Could you check a few things on this model? Use its own coordinates, in mm. Face numbers are marked on the shaded views. A direction names the side the tool comes from. Give positions to 0.01 mm unless a question says otherwise; leave off trailing zeros. Loops run counter-clockwise (first coordinate to the right, second up) from the corner with the lowest first, then second, coordinate; pieces in that order, holes last.
1. For the marked faces 1 and 2, which set-ups out of +Z, -Z, +X, -X, +Y, -Y let a thin tool reach every point of the face, with its end or its side?
2. I need wall thicknesses on line 1 along Z through (x, y) = (2.5, 0.75); line 2 along Y through (x, z) = (-2, 3.25); line 3 along Y through (x, z) = (-3.25, 1.5). Which ranges of each line are inside material? Lowest first, please.
3. For P1, Ø10, axis at y = 5, z = 2.5, coming from the +X side; P2, Ø3, axis at x = 4, y = -2.5, coming from the -Z side; P3, Ø1, axis at y = -6.5, z = 3, coming from the -X side; P4, Ø6, axis at x = 3, y = -2.5, coming from the +Z side, each with a flat end and sliding along its axis, tell me the tip position at first contact or that it passes through.
4. Imagine slicing it at A-A (z = 5.75). List the corners of the cut face in (x, y) for me, plus the area to 3 significant figures.
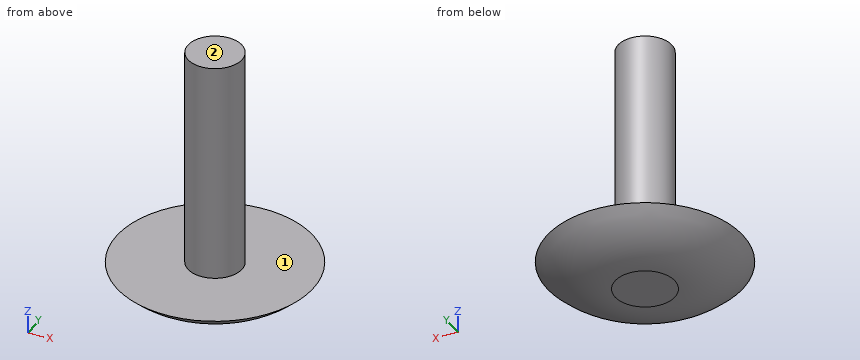
```python
from build123d import *

# Parameters (mm, degrees)
F0_R     = 9.25
F1_DEPTH = 2.7
F2_R     = 2.55
F3_DEPTH = 21


# Not quite as in the source:
# - a fillet or chamfer that OpenCascade refuses, or shapes differently, is made with other operations: its cross-section is extruded or revolved along the edge and cut away or added


with BuildPart() as f1:
    # F0 (on Top) → F1 (new body)
    with BuildSketch(Plane.XY):
        Circle(F0_R)
    extrude(amount=F1_DEPTH)

    # F2 (on face) → F3 (join)
    with BuildSketch(Plane.XY.offset(2.7)):
        Circle(F2_R)
    extrude(amount=F3_DEPTH)

    # F4: fillet of radius 9 on 1 edges, made by hand

    # F4_s1 → F4_t2 (revolve, cut)
    with BuildSketch(Plane.XZ):
        with BuildLine():
            ThreePointArc((9.25, 2.7), (6.3083994259, 0.7024099884), (2.8227144143, 0))
            Line((2.8227144143, 0), (9.25, 0))
            Line((9.25, 0), (9.25, 2.7))
        make_face()
    revolve(axis=Axis((0, 0, 0), (0, 0, 1)), mode=Mode.SUBTRACT)


solid = f1.part
```
Derived:
1. face 1: +Z
1. face 2: +Z, +X, -X, +Y, -Y
2. line 1: z = 0 to 2.7
2. line 2: y = -1.58 to 1.58
2. line 3: y = -7.09 to 7.09
3. P1: stops at x = 9.25
3. P2: stops at z = 0.01
3. P3: stops at x = -6.95
3. P4: stops at z = 23.7
4. outline: circle Ø5.1 at (0, 0)
4. area: 20.4 mm2
